Design review of the part built by this model. Coordinates are the model's own, in mm. A direction names the side the tool comes from. Coordinates: 2 decimals unless noted, no trailing zeros. Write each loop counter-clockwise with the first axis right and the second up, starting at its lowest first coordinate (ties: lowest second). Pieces come first, ordered by that corner, then holes.
Autodesk Inventor part; units mm, degrees
ref_plane "YZ Plane" through (0, 0, 0) normal (1, 0, 0) x (0, 1, 0)
ref_plane "XZ Plane" through (0, 0, 0) normal (0, 1, 0) x (-1, 0, 0)
ref_plane "XY Plane" through (0, 0, 0) normal (0, 0, 1) x (1, 0, 0)
sketch "Sketch1" plane through (0, 0, 0) normal (0, 1, 0) x (-1, 0, 0)
  point P0 (0, 0)
sketch "Sketch2" plane through (0, 0, 0) normal (0, 1, 0) x (-1, 0, 0)
  line L0 (0, 0) -> (76.2, 0)
  line L1 (76.2, 0) -> (76.2, -166.624)
  line L2 (76.2, -166.624) -> (0, -166.624)
  line L3 (0, -166.624) -> (0, 0)
  dimension "d0" = 76.2
  dimension "d1" = 166.624
extrude "Base Extrusion" add sketch "Sketch2" along normal blind 6.35
sketch "Sketch3" plane through (0, 0, 0) normal (0, 1, 0) x (-1, 0, 0)
  line L0 (76.2, 0) -> (0, 0)
  line L1 (0, 0) -> (0, -166.624)
  line L2 (0, -166.624) -> (76.2, -166.624)
  line L3 (76.2, -166.624) -> (76.2, 0)
  line L4 (10.8857, 0) -> (21.7714, 0)
  line L5 (21.7714, 0) -> (21.7714, 8.89)
  line L6 (21.7714, 8.89) -> (10.8857, 8.89)
  line L7 (10.8857, 8.89) -> (10.8857, 0)
  line L8 (32.6571, 0) -> (43.5429, 0)
  line L9 (43.5429, 0) -> (43.5429, 8.89)
  line L10 (43.5429, 8.89) -> (32.6571, 8.89)
  line L11 (32.6571, 8.89) -> (32.6571, 0)
  line L12 (54.4286, 0) -> (65.3143, 0)
  line L13 (65.3143, 0) -> (65.3143, 8.89)
  line L14 (65.3143, 8.89) -> (54.4286, 8.89)
  line L15 (54.4286, 8.89) -> (54.4286, 0)
  line L16 (76.2, -83.312) -> (0, -83.312) construction
  line L17 (76.2, -166.624) -> (0, -166.624)
  line L18 (10.8857, -166.624) -> (21.7714, -166.624)
  line L19 (21.7714, -166.624) -> (21.7714, -175.514)
  line L20 (21.7714, -175.514) -> (10.8857, -175.514)
  line L21 (10.8857, -175.514) -> (10.8857, -166.624)
  line L22 (43.5429, -166.624) -> (43.5429, -175.514)
  line L23 (43.5429, -175.514) -> (32.6571, -175.514)
  line L24 (32.6571, -175.514) -> (32.6571, -166.624)
  line L25 (32.6571, -166.624) -> (43.5429, -166.624)
  line L26 (65.3143, -166.624) -> (65.3143, -175.514)
  line L27 (65.3143, -175.514) -> (54.4286, -175.514)
  line L28 (54.4286, -175.514) -> (54.4286, -166.624)
  line L29 (54.4286, -166.624) -> (65.3143, -166.624)
  line L30 (38.1, 0) -> (38.1, -166.624) construction
  line L31 (0, -23.8034) -> (-8.89, -23.8034)
  line L32 (-8.89, -23.8034) -> (-8.89, -47.6069)
  line L33 (-8.89, -47.6069) -> (0, -47.6069)
  line L34 (0, -47.6069) -> (0, -23.8034)
  line L35 (0, -71.4103) -> (-8.89, -71.4103)
  line L36 (-8.89, -71.4103) -> (-8.89, -95.2137)
  line L37 (-8.89, -95.2137) -> (0, -95.2137)
  line L38 (0, -95.2137) -> (0, -71.4103)
  line L39 (0, -119.0171) -> (-8.89, -119.0171)
  line L40 (-8.89, -119.0171) -> (-8.89, -142.8206)
  line L41 (-8.89, -142.8206) -> (0, -142.8206)
  line L42 (0, -142.8206) -> (0, -119.0171)
  line L43 (76.2, 0) -> (76.2, -166.624)
  line L44 (76.2, -23.8034) -> (85.09, -23.8034)
  line L45 (85.09, -23.8034) -> (85.09, -47.6069)
  line L46 (85.09, -47.6069) -> (76.2, -47.6069)
  line L47 (76.2, -47.6069) -> (76.2, -23.8034)
  line L48 (76.2, -71.4103) -> (85.09, -71.4103)
  line L49 (85.09, -71.4103) -> (85.09, -95.2137)
  line L50 (85.09, -95.2137) -> (76.2, -95.2137)
  line L51 (76.2, -95.2137) -> (76.2, -71.4103)
  line L52 (76.2, -119.0171) -> (85.09, -119.0171)
  line L53 (85.09, -119.0171) -> (85.09, -142.8206)
  line L54 (85.09, -142.8206) -> (76.2, -142.8206)
  line L55 (76.2, -142.8206) -> (76.2, -119.0171)
  dimension "d4" = 10.8857
  dimension "d5" = 8.89
  dimension "d6" = 10.8857
  dimension "d7" = 10.8857
  dimension "d8" = 8.89
  dimension "d9" = 10.8857
  dimension "d10" = 8.89
  dimension "d11" = 10.8857
  dimension "d13" = 10.8857
  dimension "d14" = 76.2
  dimension "d15" = 23.8034
  dimension "d16" = 166.624
  dimension "d17" = 8.89
  dimension "d18" = 23.8034
  dimension "d19" = 8.89
  dimension "d20" = 23.8034
  dimension "d21" = 8.89
  dimension "d22" = 23.8034
  dimension "d23" = 23.8034
  dimension "d24" = 23.8034
extrude "Connections" add sketch "Sketch3" along normal blind 6.35 contours L0 L15 L14 L13 | L44 L45 L46 L3 | L0 L11 L10 L9 | L48 L49 L50 L3 | L0 L7 L6 L5 | L52 L53 L54 L3 | L1 L33 L32 L31 | L26 L27 L28 L2 | L1 L37 L36 L35 | L22 L23 L24 L2 | L1 L41 L40 L39 | L19 L20 L21 L2
sketch "Sketch5" plane through (0, 6.35, 0) normal (0, 1, 0) x (1, 0, 0)
  line L0 (-76.2, 0) -> (-65.3143, 0)
  line L1 (-65.3143, 0) -> (-65.3143, -8.89)
  line L2 (-65.3143, -8.89) -> (-54.4286, -8.89)
  line L3 (-54.4286, -8.89) -> (-54.4286, 0)
  line L4 (-54.4286, 0) -> (-43.5429, 0)
  line L5 (-43.5429, 0) -> (-43.5429, -8.89)
  line L6 (-43.5429, -8.89) -> (-32.6571, -8.89)
  line L7 (-32.6571, -8.89) -> (-32.6571, 0)
  line L8 (-32.6571, 0) -> (-21.7714, 0)
  line L9 (-21.7714, 0) -> (-21.7714, -8.89)
  line L10 (-21.7714, -8.89) -> (-10.8857, -8.89)
  line L11 (-10.8857, -8.89) -> (-10.8857, 0)
  line L12 (-10.8857, 0) -> (0, 0)
  line L13 (0, 0) -> (0, 23.8034)
  line L14 (0, 23.8034) -> (8.89, 23.8034)
  line L15 (8.89, 23.8034) -> (8.89, 47.6069)
  line L16 (8.89, 47.6069) -> (0, 47.6069)
  line L17 (0, 47.6069) -> (0, 71.4103)
  line L18 (0, 71.4103) -> (8.89, 71.4103)
  line L19 (8.89, 71.4103) -> (8.89, 95.2137)
  line L20 (8.89, 95.2137) -> (0, 95.2137)
  line L21 (0, 95.2137) -> (0, 119.0171)
  line L22 (0, 119.0171) -> (8.89, 119.0171)
  line L23 (8.89, 119.0171) -> (8.89, 142.8206)
  line L24 (8.89, 142.8206) -> (0, 142.8206)
  line L25 (0, 142.8206) -> (0, 166.624)
  line L26 (0, 166.624) -> (-10.8857, 166.624)
  line L27 (-10.8857, 166.624) -> (-10.8857, 175.514)
  line L28 (-10.8857, 175.514) -> (-21.7714, 175.514)
  line L29 (-21.7714, 175.514) -> (-21.7714, 166.624)
  line L30 (-21.7714, 166.624) -> (-32.6571, 166.624)
  line L31 (-32.6571, 166.624) -> (-32.6571, 175.514)
  line L32 (-32.6571, 175.514) -> (-43.5429, 175.514)
  line L33 (-43.5429, 175.514) -> (-43.5429, 166.624)
  line L34 (-43.5429, 166.624) -> (-54.4286, 166.624)
  line L35 (-54.4286, 166.624) -> (-54.4286, 175.514)
  line L36 (-54.4286, 175.514) -> (-65.3143, 175.514)
  line L37 (-65.3143, 175.514) -> (-65.3143, 166.624)
  line L38 (-65.3143, 166.624) -> (-76.2, 166.624)
  line L39 (-76.2, 166.624) -> (-76.2, 142.8206)
  line L40 (-76.2, 142.8206) -> (-85.09, 142.8206)
  line L41 (-85.09, 142.8206) -> (-85.09, 119.0171)
  line L42 (-85.09, 119.0171) -> (-76.2, 119.0171)
  line L43 (-76.2, 119.0171) -> (-76.2, 95.2137)
  line L44 (-76.2, 95.2137) -> (-85.09, 95.2137)
  line L45 (-85.09, 95.2137) -> (-85.09, 71.4103)
  line L46 (-85.09, 71.4103) -> (-76.2, 71.4103)
  line L47 (-76.2, 71.4103) -> (-76.2, 47.6069)
  line L48 (-76.2, 47.6069) -> (-85.09, 47.6069)
  line L49 (-85.09, 47.6069) -> (-85.09, 23.8034)
  line L50 (-85.09, 23.8034) -> (-76.2, 23.8034)
  line L51 (-76.2, 23.8034) -> (-76.2, 0)
equation "\"d5\" = WallConA"
equation "\"d6\" = -0.75 * d4 + 0.25 * d14"
equation "\"d7\" = d4"
equation "\"d8\" = d5"
equation "\"d9\" = d4"
equation "\"d10\" = d5"
equation "\"d11\" = d6"
equation "\"d13\" = d6"
equation "\"d15\" = -0.75 * d18 + 0.25 * d16"
equation "\"d17\" = WallConA"
equation "\"d18\" = 0.142857 * d16"
equation "\"d19\" = d17"
equation "\"d20\" = d18"
equation "\"d21\" = d17"
equation "\"d22\" = d18"
equation "\"d23\" = d15"
equation "\"d24\" = d15"
properties part number "Cap(Reader)"
(1) Wall thickness on line 1 (Z direction, x = 4, y = 3); line 2 (X direction, y = 3, z = -118.5); line 3 (Z direction, x = -23, y = 3.5): over which ranges is each line inside the solid? List them lowest first.
(2) Mouldability with a two-part tool opening along X and no side actions: class faces 1 (the flat face through (-27, 3, 0)), 2 (the flat face through (5, 3, -95.214)), 3 (the flat face through (-54.429, 3, 5)), 4 (the flat face through (-76.2, 3, -107)) as +X half, -X half, draft (parallel to the pull), parting line (faces both ways), or undercut.
(3) Consider section A-A (z = -54). Give the boundary of the cut face in (x, y).
(4) Insertion check: pin 1 Ø3 at (x, y) = (6.5, 3.5) entering from +Z; pin 2 Ø2 at (x, y) = (-51, 3.5) entering from -Z; pin 3 Ø1.9 at (y, z) = (3.5, -171) entering from +X. Each pin has a flat end and moves straight along its axis. Give the tip position at first contact, or say it passes through.
(5) For faces 5 (the flat face through (-32.657, 3, -171)), 6 (the flat face through (0, 3, -60)), 7 (the flat face through (-65.314, 3, 4)), 8 (the flat face through (-5, 3, 0)), 9 (the flat face through (-65.314, 3, -171)), list the 3-axis set-ups (+Z, -Z, +X, -X, +Y, -Y) from which the entire face can be reached by the end or side of a thin tool; tool diameter is ignored.
(6) Consider section B-B (x = -28.5). Give the boundary of the cut face in (y, z), plus the area to 3 significant figures.
Results:
1. line 1: z = -142.82 to -119.02, -95.21 to -71.41, -47.61 to -23.8
1. line 2: x = -76.2 to 0
1. line 3: z = -166.62 to 0
2. face 1: undercut
2. face 2: draft
2. face 3: undercut
2. face 4: -X half
3. outline: (-76.2, 0) - (0, 0) - (0, 6.35) - (-76.2, 6.35) - close
4. pin 1: stops at z = -23.8
4. pin 2: stops at z = -166.62
4. pin 3: stops at x = -10.89
5. face 5: -Z, +Y, -Y
5. face 6: +X, +Y, -Y
5. face 7: +Z, -X, +Y, -Y
5. face 8: +Z, +X, +Y, -Y
5. face 9: -Z, -X, +Y, -Y
6. outline: (0, -166.62) - (6.35, -166.62) - (6.35, 0) - (0, 0) - close
6. area: 1,060 mm2
